from build123d import *

# Parameters (mm, degrees)
SKETCH2_W           = 55
SKETCH2_H           = 90
SKETCH2_R           = 4.25
BOSS_EXTRUDE1_DEPTH = 10
FILLET1_R           = 10
CUT_EXTRUDE1_DEPTH  = 600


with BuildPart() as part:
    # Sketch2 → Boss-Extrude1 (new body)
    with BuildSketch(Plane.XY):
        with Locations((46.5, 265.320623632)):
            Rectangle(SKETCH2_W, SKETCH2_H)
        with Locations((59, 293.320623632)):
            Circle(SKETCH2_R, mode=Mode.SUBTRACT)
        with Locations((59, 248.320623632)):
            Circle(SKETCH2_R, mode=Mode.SUBTRACT)
        with BuildLine():
            Line((30, 278.070623632), (38, 278.070623632))
            ThreePointArc((38, 278.070623632), (39.414213562, 278.656410069), (40, 280.070623632))
            Line((40, 280.070623632), (40, 286.570623632))
            ThreePointArc((40, 286.570623632), (39.414213562, 287.984837194), (38, 288.570623632))
            Line((38, 288.570623632), (30, 288.570623632))
            ThreePointArc((30, 288.570623632), (28.585786438, 287.984837194), (28, 286.570623632))
            Line((28, 286.570623632), (28, 280.070623632))
            ThreePointArc((28, 280.070623632), (28.585786438, 278.656410069), (30, 278.070623632))
        make_face(mode=Mode.SUBTRACT)
        with BuildLine():
            Line((30, 233.070623632), (38, 233.070623632))
            ThreePointArc((38, 233.070623632), (39.414213562, 233.656410069), (40, 235.070623632))
            Line((40, 235.070623632), (40, 241.570623632))
            ThreePointArc((40, 241.570623632), (39.414213562, 242.984837194), (38, 243.570623632))
            Line((38, 243.570623632), (30, 243.570623632))
            ThreePointArc((30, 243.570623632), (28.585786438, 242.984837194), (28, 241.570623632))
            Line((28, 241.570623632), (28, 235.070623632))
            ThreePointArc((28, 235.070623632), (28.585786438, 233.656410069), (30, 233.070623632))
        make_face(mode=Mode.SUBTRACT)
    extrude(amount=BOSS_EXTRUDE1_DEPTH)

    # Fillet1
    fillet1_edges = [part.edges().sort_by_distance(p)[0] for p in [
        (74, 220.320623632, 5),
        (19, 220.320623632, 5),
        (19, 310.320623632, 5),
        (74, 310.320623632, 5),
    ]]
    fillet(fillet1_edges, radius=FILLET1_R)

    # Sketch4 → Cut-Extrude1 (cut)
    with BuildSketch(Plane(origin=(-127, 1084.797720172, -1205.109910301), x_dir=(0, 1, 0), z_dir=(-1, 0, 0))):
        Polygon((-781.47709654, -1215.209910301), (-501.47709654, -1215.209910301), (-501.47709654, -743.209910301), (-781.47709654, -743.2099103), align=None)
        with BuildLine():
            Line((-206.47709654, -743.209910301), (-96.47709654, -743.209910301))
            ThreePointArc((-96.47709654, -743.209910301), (-89.406028728, -746.138842489), (-86.47709654, -753.209910301))
            Line((-86.47709654, -753.209910301), (-86.47709654, -1205.209910301))
            ThreePointArc((-86.47709654, -1205.209910301), (-89.406028728, -1212.280978113), (-96.47709654, -1215.209910301))
            Line((-96.47709654, -1215.209910301), (-206.47709654, -1215.209910301))
            ThreePointArc((-206.47709654, -1215.209910301), (-213.548164352, -1212.280978113), (-216.47709654, -1205.209910301))
            Line((-216.47709654, -1205.209910301), (-216.47709654, -753.209910301))
            ThreePointArc((-216.47709654, -753.209910301), (-213.548164352, -746.138842489), (-206.47709654, -743.209910301))
        make_face()
    extrude(amount=-CUT_EXTRUDE1_DEPTH, mode=Mode.SUBTRACT)


solid = part.part
Source: CAD feature listing. Evaluate the final solid. Frame: model axes, mm. A direction names the side the tool comes from. Give positions to 0.01 mm unless a question says otherwise; leave off trailing zeros. Write each loop counter-clockwise with the first axis right and the second up, starting at its lowest first coordinate (ties: lowest second). Pieces come first, ordered by that corner, then holes. Notation, with made-up numbers: (49.25, -12.75) -> (60.25, -12.75) arc R10 cw to (60.25, 1.25) -> close; hole circle Ø3 at (50, 5). An arc over 180 degrees is marked (long way). Return JSON: item names as keys, results as strings. Group by question number.
1. Section A-A, the plane y = 283.5. Output: boundary loops of the cut face in (x, z).
2. Material intervals for line 1 (Y direction, x = 33, z = 2); line 2 (X direction, y = 284.5, z = 3.5); line 3 (X direction, y = 246, z = 6.5), sorted ascending. Write a range as from..to.
3. Mould query, pull axis Y, two halves, no side actions, for faces 1 (the face through (34, 233.071, 5)), 2 (the face through (21.85, 223.33, 5.07)), 3 (the face through (39.4, 233.64, 4.93)), 4 (the face through (73.88, 301.86, 5.07)). Classes: +Y half, -Y half, draft (parallel to the pull), parting line (faces both ways), or undercut.
4. Pin query (flat end, axial travel): pin 1 Ø5 at (x, y) = (58.5, 293.5) entering from -Z. Return the tip coordinate at first contact, or that it passes through.
5. Section D-D, the plane x = 70. Output: boundary loops of the cut face in (y, z), then the cut area to 3 significant figures.
6. Access query for faces 5 (the face through (28.57, 233.67, 4.93)), 6 (the face through (46, 303.321, 5)). Directions: +Z, -Z, +X, -X, +Y, -Y. A direction counts if a zero-diameter tool reaches every point of the face in a straight line with its end or side. Return the directions, or none.
7. Section B-B, the plane x = 59. Output: boundary loops of the cut face in (y, z), then the cut area to 3 significant figures.
8. Section C-C, the plane z = 3. Output: boundary loops of the cut face in (x, y), then the cut area to 3 significant figures.
Determined:
{
 "1": {"outline": "(19, 0) -> (28, 0) -> (28, 10) -> (19, 10) -> close; (40, 0) -> (74, 0) -> (74, 10) -> (40, 10) -> close"},
 "2": {"line 1": "y = 220.32..233.07, 243.57..278.07, 288.57..303.32", "line 2": "x = 19..28, 40..74", "line 3": "x = 19..55.44, 62.56..74"},
 "3": {"face 1": "undercut", "face 2": "-Y half", "face 3": "undercut", "face 4": "+Y half"},
 "4": {"pin 1": "passes through"},
 "5": {"outline": "(222.32, 0) -> (303.32, 0) -> (303.32, 10) -> (222.32, 10) -> close", "area": "810 mm2"},
 "6": {"face 5": "+Z, -Z", "face 6": "+Z, -Z, +X, -X, +Y"},
 "7": {"outline": "(220.32, 0) -> (244.07, 0) -> (244.07, 10) -> (220.32, 10) -> close; (252.57, 0) -> (289.07, 0) -> (289.07, 10) -> (252.57, 10) -> close; (297.57, 0) -> (303.32, 0) -> (303.32, 10) -> (297.57, 10) -> close", "area": "660 mm2"},
 "8": {"outline": "(19, 230.32) arc R10 ccw to (29, 220.32) -> (64, 220.32) arc R10 ccw to (74, 230.32) -> (74, 300.32) arc R10 ccw to (73.54, 303.32) -> (19.46, 303.32) arc R10 ccw to (19, 300.32) -> close; hole (28, 235.07) arc R2 ccw to (30, 233.07) -> (38, 233.07) arc R2 ccw to (40, 235.07) -> (40, 241.57) arc R2 ccw to (38, 243.57) -> (30, 243.57) arc R2 ccw to (28, 241.57) -> close; hole (28, 280.07) arc R2 ccw to (30, 278.07) -> (38, 278.07) arc R2 ccw to (40, 280.07) -> (40, 286.57) arc R2 ccw to (38, 288.57) -> (30, 288.57) arc R2 ccw to (28, 286.57) -> close; hole circle Ø8.5 at (59, 248.32); hole circle Ø8.5 at (59, 293.32)", "area": "4,160 mm2"}
}
